Geometry check sheet. Reference: the model listing, model coordinates, mm. Face numbers are marked on the shaded views. A direction names the side the tool comes from. Coordinates: 2 decimals unless noted, no trailing zeros. Write each loop counter-clockwise with the first axis right and the second up, starting at its lowest first coordinate (ties: lowest second). Pieces come first, ordered by that corner, then holes.
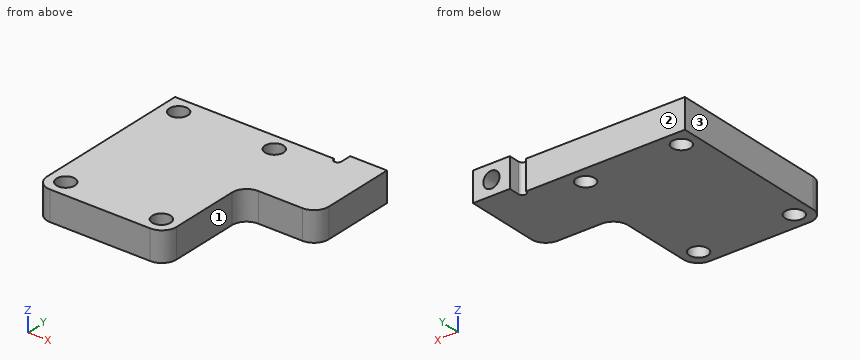
Autodesk Inventor part; units mm, degrees
ref_plane "作業平面1" through (0, 0, 0) normal (0, 0, 1) x (1, 0, 0)
ref_plane "YZ Plane" through (0, 0, 0) normal (1, 0, 0) x (0, 1, 0)
ref_plane "XZ Plane" through (0, 0, 0) normal (0, 1, 0) x (-1, 0, 0)
ref_plane "作業平面1" through (0, 0, 0) normal (0, 0, 1) x (1, 0, 0)
sketch "スケッチ1" plane through (0, 0, 0) normal (0, 0, 1) x (1, 0, 0)
  line L0 (0, -24) -> (-27.3, -24)
  line L1 (-3.7, -24) -> (-3.7, -10.5)
  line L2 (-3.7, -10.5) -> (6.3, -10.5)
  line L3 (6.3, -10.5) -> (6.3, 1.5)
  line L4 (6.3, 1.5) -> (1.3, 1.5)
  line L5 (-27.3, 0) -> (0, 0)
  line L6 (1.3, 1.5) -> (1.3, 0)
  circle A0 centre (-6, -21.7) radius 1.25
  circle A1 centre (-19, -21.7) radius 1.25
  circle A2 centre (-6, -21.7) radius 2.3 construction
  circle A3 centre (-19, -21.7) radius 2.3 construction
  line L7 (1.3, 0) -> (0, 0)
  line L8 (-21.3, -24) -> (-21.3, 0)
  circle A4 centre (-6, -2.3) radius 1.25
  circle A5 centre (-19, -2.3) radius 1.25
  line L9 (1.3, 0) -> (0.8, 0)
  arc A6 (0.3, 0) -> (1.3, 0) centre (0.8, 0) ccw
  dimension "d0" = 1.5
  dimension "d1" = 12
  dimension "d2" = 10
  dimension "d3" = 5
  dimension "d9" = 0.5
extrude "押し出し1" add sketch "スケッチ1" along normal blind 4 contours L0 L8 L5 L7 A6 L6 L4 L3 L2 L1
sketch "スケッチ2" plane through (1.3, 1.5, 0) normal (0, 1, 0) x (1, 0, 0)
  line L0 (5, 0) -> (5, -4)
  line L1 (0, 0) -> (-22.6, 0)
  line L2 (5, -4) -> (0, 0) construction
  circle A0 centre (2.5, -2) radius 1.1
  point P0 (-1.3, 0)
  dimension "d6" = 2.2
extrude "押し出し2" cut sketch "スケッチ2" against normal blind 5
fillet "フィレット1" radius 2 4 edges at (6.3, -10.5, 2) (-3.7, -10.5, 2) (-3.7, -24, 2) (-21.3, -24, 2)
properties part number "SolenoidMount"
1. Sectioned sample at C-C, the plane x = -1.25. Record the boundary of the cut face in (y, z), and give its area (3 significant figures).
Computed values:
outline: (-10.5, 0) - (0, 0) - (0, 4) - (-10.5, 4) - close
area: 42.0 mm2
2. Sectioned sample at A-A, the plane z = 0.55. Record the boundary of the cut face in (x, y), and give its area (3 significant figures).
Computed values:
outline: (-21.3, -22) arc R2 ccw to (-19.3, -24) - (-5.7, -24) arc R2 ccw to (-3.7, -22) - (-3.7, -12.5) arc R2 cw to (-1.7, -10.5) - (4.3, -10.5) arc R2 ccw to (6.3, -8.5) - (6.3, 1.5) - (1.3, 1.5) - (1.3, 0) arc R0.5 cw to (0.3, 0) - (-21.3, 0) - close; hole circle Ø2.5 at (-19, -21.7); hole circle Ø2.5 at (-19, -2.3); hole circle Ø2.5 at (-6, -21.7); hole circle Ø2.5 at (-6, -2.3)
area: 513 mm2
3. Sectioned sample at B-B, the plane x = -6.5. Record the boundary of the cut face in (y, z), and give its area (3 significant figures).
Computed values:
outline: (-24, 0) - (-22.85, 0) - (-22.85, 4) - (-24, 4) - close; (-20.55, 0) - (-3.45, 0) - (-3.45, 4) - (-20.55, 4) - close; (-1.15, 0) - (0, 0) - (0, 4) - (-1.15, 4) - close
area: 77.7 mm2
4. Thickness scan on line 1 along Y through (x, z) = (-6.5, 2.6); line 2 along Y through (x, z) = (-18, 1.9); line 3 along X through (y, z) = (-1.2, 2). Record the ranges inside material, lowest first.
Computed values:
line 1: y = -24 to -22.85, -20.55 to -3.45, -1.15 to 0
line 2: y = -24 to -22.45, -20.95 to -3.05, -1.55 to 0
line 3: x = -21.3 to -19.59, -18.41 to -6.59, -5.41 to 2.7, 4.9 to 6.3
5. Sectioned sample at D-D, the plane z = 2. Record the boundary of the cut face in (x, y), and give its area (3 significant figures).
Computed values:
outline: (-21.3, -22) arc R2 ccw to (-19.3, -24) - (-5.7, -24) arc R2 ccw to (-3.7, -22) - (-3.7, -12.5) arc R2 cw to (-1.7, -10.5) - (4.3, -10.5) arc R2 ccw to (6.3, -8.5) - (6.3, 1.5) - (4.9, 1.5) - (4.9, -3.5) - (2.7, -3.5) - (2.7, 1.5) - (1.3, 1.5) - (1.3, 0) arc R0.5 cw to (0.3, 0) - (-21.3, 0) - close; hole circle Ø2.5 at (-19, -21.7); hole circle Ø2.5 at (-19, -2.3); hole circle Ø2.5 at (-6, -21.7); hole circle Ø2.5 at (-6, -2.3)
area: 502 mm2
6. Gauge pin test, flat ends, axial feed: pin 1 Ø1 at (x, z) = (-17, 3) entering from +Y; pin 2 Ø2 at (y, z) = (-15.5, 1) entering from +X. Record the tip position at first contact, or that the pin passes through.
Computed values:
pin 1: stops at y = 0
pin 2: stops at x = -3.7
7. Access from +Z, -Z, +X, -X, +Y, -Y to the whole of each face (thin tool, end or side, straight path). Record for the marked faces 1, 2 and 3.
Computed values:
face 1: +Z, -Z, +X, -Y
face 2: +Z, -Z, -X, +Y
face 3: +Z, -Z, -X, +Y, -Y
